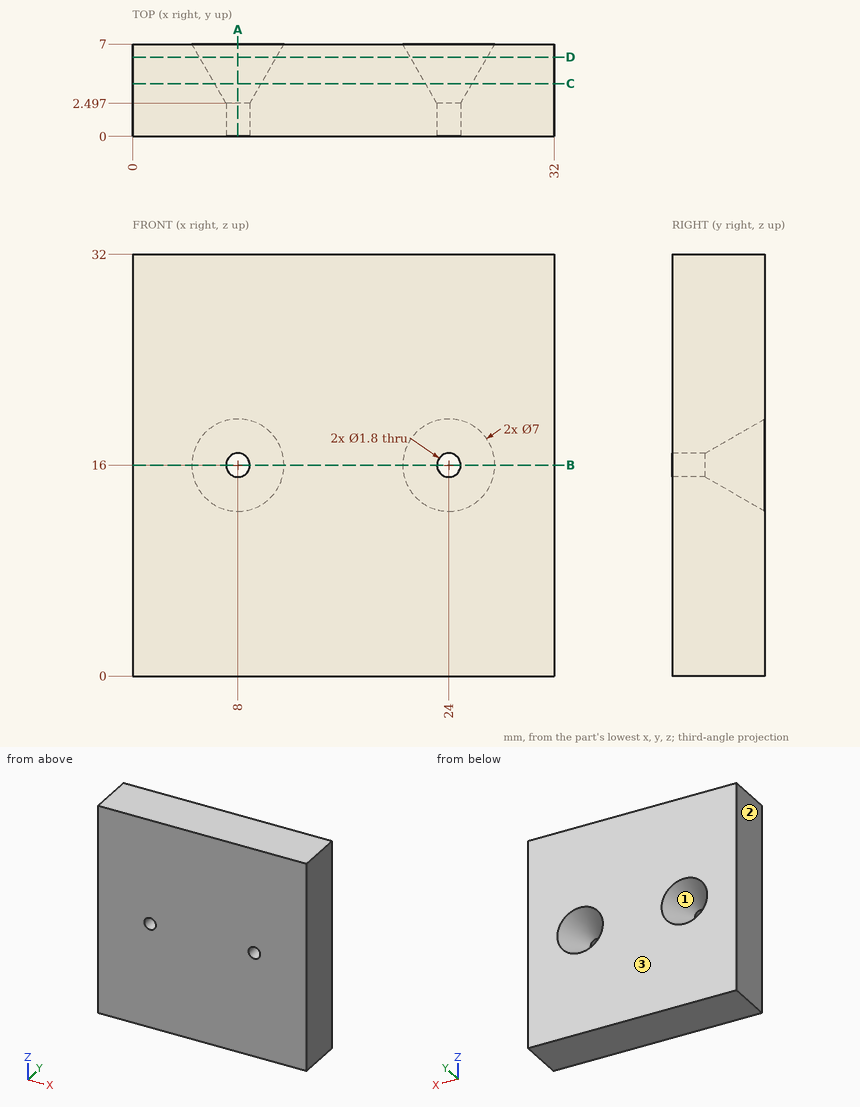
Geometry check sheet. Reference: drawing and pictorial views, mm from the part's lowest x, y, z. Round coordinates to 2 decimals unless told otherwise and drop trailing zeros. Loops run counter-clockwise (first coordinate to the right, second up) from the corner with the lowest first, then second, coordinate; pieces in that order, holes last. Notation, with made-up numbers: (-1, -15.5) - (6, -15.5) arc R21 ccw to (6, 15.5) - close; hole circle Ø10 at (73.5, 38). An arc over 180 degrees is marked (long way). Answer in a Markdown table with one row per item. Add a question column.
Q1. Section check D-D on y = 6. Enter the section's corners in (x, z) (1 decimal).
Q2. Section check C-C on y = 4. Enter the section's corners in (x, z), plus the area to 3 significant figures.
Q3. Release check for a two-part mould opening along X. For the marked faces 1, 2 and 3 record: pulls with the +X half, pulls with the -X half, needs draft (parallel to the pull), parting line crosses it, or undercut.
Q4. Section check A-A on x = 8. Enter the section's corners in (y, z).
Q5. Section check B-B on z = 16. Enter the section's corners in (x, y), plus the area to 3 significant figures.
Q6. Gauge pin test, flat end, axial feed: pin 1 (2 mm diameter, centred on x = 8, z = 16, fed in from +Y). Record the tip position at first contact, or that the pin passes through.
Q7. Material ranges on line 1 (X direction, y = 1.75, z = 16); line 2 (Z direction, x = 24, y = 0.85); line 3 (X direction, y = 6.25, z = 16), recorded low to high.
Found:
| question | item | result |
|---|---|---|
| 1 | outline | (0, 0) - (32, 0) - (32, 32) - (0, 32) - close; hole circle Ø5.8 at (8, 16); hole circle Ø5.8 at (24, 16) |
| 2 | outline | (0, 0) - (32, 0) - (32, 32) - (0, 32) - close; hole circle Ø3.54 at (8, 16); hole circle Ø3.54 at (24, 16) |
| 2 | area | 1,000 mm² |
| 3 | face 1 | undercut |
| 3 | face 2 | pulls with the -X half |
| 3 | face 3 | needs draft |
| 4 | outline | (0, 0) - (7, 0) - (7, 12.5) - (2.5, 15.1) - (0, 15.1) - close; (0, 16.9) - (2.5, 16.9) - (7, 19.5) - (7, 32) - (0, 32) - close |
| 5 | outline | (0, 0) - (7.1, 0) - (7.1, 2.5) - (4.5, 7) - (0, 7) - close; (8.9, 0) - (23.1, 0) - (23.1, 2.5) - (20.5, 7) - (11.5, 7) - (8.9, 2.5) - close; (24.9, 0) - (32, 0) - (32, 7) - (27.5, 7) - (24.9, 2.5) - close |
| 5 | area | 175 mm² |
| 6 | pin 1 | stops at y = 2.67 |
| 7 | line 1 | x = 0 to 7.1, 8.9 to 23.1, 24.9 to 32 |
| 7 | line 2 | z = 0 to 15.1, 16.9 to 32 |
| 7 | line 3 | x = 0 to 4.93, 11.07 to 20.93, 27.07 to 32 |
